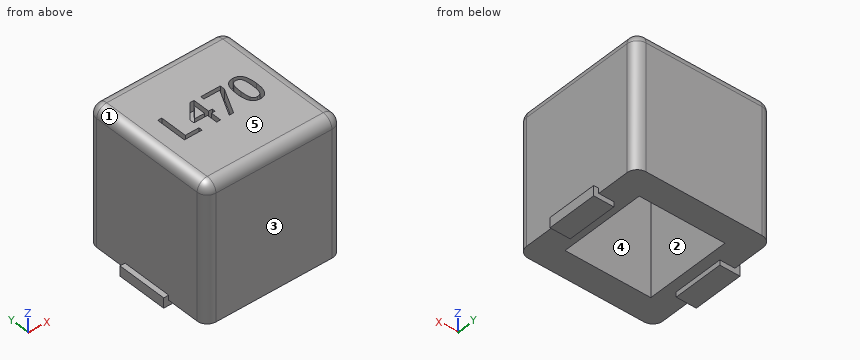
Autodesk Inventor part; units mm, degrees
ref_plane "YZ Plane" through (0, 0, 0) normal (1, 0, 0) x (0, 1, 0)
ref_plane "XZ Plane" through (0, 0, 0) normal (0, 1, 0) x (-1, 0, 0)
ref_plane "XY Plane" through (0, 0, 0) normal (0, 0, 1) x (1, 0, 0)
sketch "Sketch2" plane through (0, 0, 0) normal (0, 0, 1) x (1, 0, 0)
  line L0 (-6.75, -6.75) -> (6.75, -6.75)
  line L1 (6.75, -6.75) -> (6.75, 6.75)
  line L2 (6.75, 6.75) -> (-6.75, 6.75)
  line L3 (-6.75, 6.75) -> (-6.75, -6.75)
  line L4 (-6.75, -6.75) -> (6.75, 6.75) construction
  line L5 (6.75, -6.75) -> (-6.75, 6.75) construction
  line L6 (-6.75, -6.75) -> (6.75, -6.75) construction
  line L7 (6.75, -6.75) -> (6.75, -2.5) construction
  line L8 (6.75, -2.5) -> (-6.75, -2.5) construction
  line L9 (-6.75, -2.5) -> (-6.75, -6.75) construction
  line L10 (-7.25, -2.5) -> (7.25, -2.5)
  line L11 (7.25, -2.5) -> (7.25, 2.5)
  line L12 (7.25, 2.5) -> (-7.25, 2.5)
  line L13 (-7.25, 2.5) -> (-7.25, -2.5)
  line L14 (-7.25, 2.5) -> (-5.25, 2.5)
  line L15 (-5.25, 2.5) -> (-5.25, -2.5)
  line L16 (-5.25, -2.5) -> (-7.25, -2.5)
  line L17 (-7.25, -2.5) -> (-7.25, 2.5)
  line L18 (7.25, 2.5) -> (5.25, 2.5)
  line L19 (5.25, 2.5) -> (5.25, -2.5)
  line L20 (5.25, -2.5) -> (7.25, -2.5)
  line L21 (7.25, -2.5) -> (7.25, 2.5)
  line L22 (4.25, -4.25) -> (-4.25, -4.25)
  line L23 (-4.25, -4.25) -> (-4.25, 4.25)
  line L24 (-4.25, 4.25) -> (4.25, 4.25)
  line L25 (4.25, 4.25) -> (4.25, -4.25)
  line L26 (4.25, -4.25) -> (-4.25, 4.25) construction
  line L27 (-4.25, -4.25) -> (4.25, 4.25) construction
  point P0 (0, 0)
  point P1 (0, -2.5)
  point P2 (-6.75, 2.5)
  point P3 (6.75, -2.5)
  point P4 (6.75, 2.5)
  dimension "d2" = 13.5
  dimension "d4" = 4.25
  dimension "d5" = 5
  dimension "d6" = 0.5
  dimension "d7" = 0.5
  dimension "d8" = 2
  dimension "d9" = 2
  dimension "d16" = 8.5
extrude "Extrusion2" add sketch "Sketch2" along normal blind 13.5 contours L3 L10 L23 L22 L25 L1 L0 | L3 L12 L15 L10 | L10 L19 L12 L1 | L3 L2 L1 L12 L25 L24 L23 | L15 L12 L23 L10 | L10 L25 L12 L19 | L23 L12 L25 L10 | L10 L25 L22 L23 | L23 L24 L25 L12
extrude "Extrusion3" add sketch "Sketch2" against normal blind 0.5 contours L3 L12 L15 L10 | L10 L19 L12 L1
extrude "Extrusion4" add sketch "Sketch2" along normal mid plane 1 contours L10 L13 L12 L3 | L1 L12 L11 L10
extrude "Extrusion5" cut sketch "Sketch2" along normal blind 10 contours L23 L12 L25 L10 | L10 L25 L22 L23 | L23 L24 L25 L12
sketch "Sketch3" plane through (0, 0, 13.5) normal (0, 0, 1) x (1, 0, 0)
  line L0 (-4.532, 1.7426) -> (3.9775, 1.7426) construction
  line L1 (3.9775, 1.7426) -> (3.9775, -2.8625) construction
  line L2 (3.9775, -2.8625) -> (-4.532, -2.8625) construction
  line L3 (-4.532, -2.8625) -> (-4.532, 1.7426) construction
  line L4 (-2.4572, -1.3672) -> (-4.2232, -1.3672)
  line L5 (-4.2232, -1.3672) -> (-4.2232, 1.6808)
  line L6 (-4.2232, 1.6808) -> (-3.8182, 1.6808)
  line L7 (-3.8182, 1.6808) -> (-3.8182, -1.0065)
  line L8 (-3.8182, -1.0065) -> (-2.4572, -1.0065)
  line L9 (-2.4572, -1.0065) -> (-2.4572, -1.3672)
  line L10 (-0.2638, -0.3199) -> (-0.6269, -0.3199)
  line L11 (-0.6269, -0.3199) -> (-0.6269, -1.3672)
  line L12 (-0.6269, -1.3672) -> (-1.0196, -1.3672)
  line L13 (-1.0196, -1.3672) -> (-1.0196, -0.3199)
  line L14 (-1.0196, -0.3199) -> (-2.3658, -0.3199)
  line L15 (-2.3658, -0.3199) -> (-2.3658, 0.1099)
  line L16 (-2.3658, 0.1099) -> (-1.0023, 1.6808)
  line L17 (-1.0023, 1.6808) -> (-0.6269, 1.6808)
  line L18 (-0.6269, 1.6808) -> (-0.6269, 0.0086)
  line L19 (-0.6269, 0.0086) -> (-0.2638, 0.0086)
  line L20 (-0.2638, 0.0086) -> (-0.2638, -0.3199)
  line L21 (-1.0196, 0.0086) -> (-1.0196, 1.1992)
  line L22 (-1.0196, 1.1992) -> (-2.0447, 0.0086)
  line L23 (-2.0447, 0.0086) -> (-1.0196, 0.0086)
  line L24 (1.9765, 1.2239) -> (0.6575, -1.3672)
  line L25 (0.6575, -1.3672) -> (0.2228, -1.3672)
  line L26 (0.2228, -1.3672) -> (1.6159, 1.3227)
  line L27 (1.6159, 1.3227) -> (0.0425, 1.3227)
  line L28 (0.0425, 1.3227) -> (0.0425, 1.6808)
  line L29 (0.0425, 1.6808) -> (1.9765, 1.6808)
  line L30 (1.9765, 1.6808) -> (1.9765, 1.2239)
  spline S0 degree 2 poles (4.2464, 0.1568) (4.2464, -0.6632) (3.7697, -1.4314) (3.2733, -1.4314) knots 0 0 0 1 2 2 2
  spline S1 degree 2 poles (3.2733, -1.4314) (2.7694, -1.4314) (2.2976, -0.6484) (2.2976, 0.1544) knots 0 0 0 1 2 2 2
  spline S2 degree 2 poles (2.2976, 0.1544) (2.2976, 0.9794) (2.7743, 1.7426) (3.2733, 1.7426) knots 0 0 0 1 2 2 2
  spline S3 degree 2 poles (3.2733, 1.7426) (3.7747, 1.7426) (4.2464, 0.9522) (4.2464, 0.1568) knots 0 0 0 1 2 2 2
  spline S4 degree 2 poles (3.7228, -0.7719) (3.7821, -0.6212) (3.8315, -0.1569) (3.8315, 0.1568) knots 0 0 0 1 2 2 2
  spline S5 degree 2 poles (3.8315, 0.1568) (3.8315, 0.4705) (3.7821, 0.9324) (3.7203, 1.088) knots 0 0 0 1 2 2 2
  spline S6 degree 2 poles (3.7203, 1.088) (3.6586, 1.2436) (3.4437, 1.4042) (3.2733, 1.4042) knots 0 0 0 1 2 2 2
  spline S7 degree 2 poles (3.2733, 1.4042) (3.1028, 1.4042) (2.883, 1.2436) (2.8188, 1.0831) knots 0 0 0 1 2 2 2
  spline S8 degree 2 poles (2.8188, 1.0831) (2.757, 0.9275) (2.7126, 0.4532) (2.7126, 0.1544) knots 0 0 0 1 2 2 2
  spline S9 degree 2 poles (2.7126, 0.1544) (2.7126, -0.1667) (2.7521, -0.5965) (2.8163, -0.7645) knots 0 0 0 1 2 2 2
  spline S10 degree 2 poles (2.8163, -0.7645) (2.8756, -0.9226) (3.0954, -1.093) (3.2733, -1.093) knots 0 0 0 1 2 2 2
  spline S11 degree 2 poles (3.2733, -1.093) (3.4412, -1.093) (3.6611, -0.9324) (3.7228, -0.7719) knots 0 0 0 1 2 2 2
  point P0 (0, 0)
fillet "Fillet1" radius 1 8 edges at (0, 6.75, 13.5) (-6.75, 0, 13.5) (0, -6.75, 13.5) (6.75, 0, 13.5) (-6.75, 6.75, 6.75) (-6.75, -6.75, 6.75) (6.75, 6.75, 6.75) (6.75, -6.75, 6.75)
extrude "Extrusion7" cut sketch "Sketch3" against normal blind 1
properties part number "SINC1313-470_L470_SMD_3DPrint"
Part model, mm, in its own coordinate system. Face numbers are marked on the shaded views. A direction names the side the tool comes from. Give positions to 0.01 mm unless a question says otherwise; leave off trailing zeros. Write each loop counter-clockwise with the first axis right and the second up, starting at its lowest first coordinate (ties: lowest second). Pieces come first, ordered by that corner, then holes.
1) Probe L1, parallel to X at y = 0.25, z = 9.5; L2, parallel to Z at x = 2.75, y = 1.5. List the from-to ranges inside material, lowest first.
Resolved:
L1: x = -6.75 to -4.25, 4.25 to 6.75
L2: z = 10 to 12.5
2) Cut at B-B on y = -2.25. Write the cut outline in (x, z), then the cut area to 3 significant figures.
Resolved:
outline: (-7.25, -0.5) - (-5.25, -0.5) - (-5.25, 0) - (-4.25, 0) - (-4.25, 10) - (4.25, 10) - (4.25, 0) - (5.25, 0) - (5.25, -0.5) - (7.25, -0.5) - (7.25, 0.5) - (6.75, 0.5) - (6.75, 12.5) arc R1 ccw to (5.75, 13.5) - (-5.75, 13.5) arc R1 ccw to (-6.75, 12.5) - (-6.75, 0.5) - (-7.25, 0.5) - close
area: 99.3 mm2
3) Two-plate mould, pull along Y, no slides. Class the marked faces 3, 4 and 5: released by +Y, released by -Y, zero draft, split by the parting line, or undercut.
Resolved:
face 3: released by -Y
face 4: undercut
face 5: zero draft
4) Cut at D-D on z = 7.5. Write the cut outline in (x, y), then the cut area to 3 significant figures.
Resolved:
outline: (-6.75, -5.75) arc R1 ccw to (-5.75, -6.75) - (5.75, -6.75) arc R1 ccw to (6.75, -5.75) - (6.75, 5.75) arc R1 ccw to (5.75, 6.75) - (-5.75, 6.75) arc R1 ccw to (-6.75, 5.75) - close; hole (-4.25, -4.25) - (4.25, -4.25) - (4.25, 4.25) - (-4.25, 4.25) - close
area: 109 mm2
5) Cut at A-A on z = 10.75. Write the cut outline in (x, y), then the cut area to 3 significant figures.
Resolved:
outline: (-6.75, -5.75) arc R1 ccw to (-5.75, -6.75) - (5.75, -6.75) arc R1 ccw to (6.75, -5.75) - (6.75, 5.75) arc R1 ccw to (5.75, 6.75) - (-5.75, 6.75) arc R1 ccw to (-6.75, 5.75) - close
area: 181 mm2
6) Cut at C-C on x = 5. Write the cut outline in (y, z).
Resolved:
outline: (-6.75, 0) - (6.75, 0) - (6.75, 12.5) arc R1 ccw to (5.75, 13.5) - (-5.75, 13.5) arc R1 ccw to (-6.75, 12.5) - close
7) Which spindle directions (+Z, -Z, +X, -X, +Y, -Y) get a long thin tool onto all of the face, cutting with end or side? Do the marked faces 1 and 2. Say none if no direction does.
Resolved:
face 1: +Z, -X, +Y, -Y
face 2: -Z
8) Pin check, flat tips, straight feed: pin 1 (1.1 mm diameter, centred on y = 0.5, z = 13, fed in from +X); pin 2 (0.5 mm diameter, centred on y = 0, z = 13, fed in from -X); pin 3 (0.8 mm diameter, centred on x = -3, z = 13, fed in from -Y) (3 decimals). Stop position of each tip, or through.
Resolved:
pin 1: stops at x = 6.75
pin 2: stops at x = -6.72
pin 3: stops at y = -6.745
